Can you work these out from the model? Positions are in its coordinate system, mm. A direction names the side the tool comes from. Give positions to 0.01 mm unless a question says otherwise; leave off trailing zeros. Write each loop counter-clockwise with the first axis right and the second up, starting at its lowest first coordinate (ties: lowest second). Pieces come first, ordered by that corner, then holes.
```python
from build123d import *

# Parameters (mm, degrees)
F0_R     = 3.875
F1_DEPTH = 3
F0_R_2   = 7
F2_DEPTH = 0.6
F0_R_3   = 11.5
F3_DEPTH = 2
F4_DEPTH = 2
F6_T     = 1


# Not quite as in the source:
# - a shell that OpenCascade refuses in one call is made with other operations: the cavity is built on its own and cut out
# - the program builds the solid bodies; features that only make, move or delete a surface that nothing else refers to are left out


with BuildPart() as f1:
    # F0 (on Top) → F1 (new body)
    with BuildSketch(Plane.XY):
        Circle(F0_R)
    extrude(amount=F1_DEPTH)

    # F0 (on Top) → F2 (join)
    with BuildSketch(Plane.XY):
        Circle(F0_R_2)
        Circle(F0_R, mode=Mode.SUBTRACT)
    extrude(amount=F2_DEPTH)

    # F0 (on Top) → F3 (join)
    with BuildSketch(Plane.XY):
        Circle(F0_R_3)
        Circle(F0_R_2, mode=Mode.SUBTRACT)
        Circle(F0_R_2)
        Circle(F0_R, mode=Mode.SUBTRACT)
    extrude(amount=-F3_DEPTH)

    # F0 (on Top) → F4 (join)
    with BuildSketch(Plane.XY):
        Circle(F0_R)
    extrude(amount=-F4_DEPTH)

    # F6: shell of thickness 1, made by hand


with BuildPart() as f6_core1:
    # F6_t2: copy of F1
    add(f1.part)

    # the walls: a layer under each face that stays
    f6_faces = [f6_core1.faces().sort_by_distance(p)[0] for p in [
        (-3.875, 0, 1.8),
        (-4.6666666667, -4.6666666667, 0.6),
        (-7, 0, 0.3),
        (-7.6666666667, -7.6666666667, 0),
        (-11.5, 0, -1),
        (0, 0, -2),
    ]]
    thicken(f6_faces, amount=-F6_T, mode=Mode.SUBTRACT)

    # F6_s3 → F6_t4 (revolve, cut)
    with BuildSketch(Plane.XZ):
        Polygon((3.885, 0.61), (2.875, 0.6), (2.875, -0.4), (3.875, -0.4), align=None)
    revolve(axis=Axis((0, 0, 0.6), (0, 0, 1)), mode=Mode.SUBTRACT)

    # F6_s5 → F6_t6 (revolve, cut)
    with BuildSketch(Plane.XZ):
        Polygon((7.01, 0.01), (6, 0), (6, -1), (7, -1), align=None)
    revolve(axis=Axis((0, 0, 0), (0, 0, 1)), mode=Mode.SUBTRACT)


with BuildPart() as f1_1:
    add(f1.part)

    # what is left inside the walls is the cavity
    f6_cavity = [f6_core1.part.solids().sort_by_distance(p)[0] for p in [
        (0, -2, -0.99),
    ]]
    add(f6_cavity, mode=Mode.SUBTRACT)


solid = f1_1.part
```
1) Suppose I cut it at A-A on x = 0. Write out the boundary of the cut face in (y, z) (3 decimals), plus the area to 4 significant figures.
Values follow:
outline: (-11.5, -2) - (11.5, -2) - (11.5, 0) - (7, 0) - (7, 0.6) - (3.875, 0.6) - (3.875, 3) - (2.875, 3) - (2.875, -0.4) - (6, -0.4) - (6, -1) - (-6, -1) - (-6, -0.4) - (-2.875, -0.4) - (-2.875, 3) - (-3.875, 3) - (-3.875, 0.6) - (-7, 0.6) - (-7, 0) - (-11.5, 0) - close
area: 46.25 mm2
2) Suppose I cut it at C-C on z = 1.7. Write out the boundary of the cut face in (x, y) (3 decimals), plus the area to 3 significant figures.
Values follow:
outline: circle Ø7.75 at (0, 0); hole circle Ø5.75 at (0, 0)
area: 21.2 mm2
3) For faces 1 (the face through (-1, 3, 3)), 2 (the face through (6.466, -2.681, 0.296)), 3 (the face through (0, 0, -1)), which set-ups out of +Z, -Z, +X, -X, +Y, -Y let a thin tool reach every point of the face, with its end or its side?
Values follow:
face 1: +Z, +X, -X, +Y, -Y
face 2: +Z
face 3: none
4) Suppose I cut it at B-B on y = 5. Write out the boundary of the cut face in (x, z), plus the area to 3 significant figures.
Values follow:
outline: (-10.36, -2) - (10.36, -2) - (10.36, 0) - (4.9, 0) - (4.9, 0.6) - (-4.9, 0.6) - (-4.9, 0) - (-10.36, 0) - close; hole (-3.32, -1) - (3.32, -1) - (3.32, -0.4) - (-3.32, -0.4) - close
area: 43.3 mm2
5) For pin 1 Ø1.5 at (x, z) = (2.5, -0.5) entering from +Y; pin 2 Ø2 at (x, y) = (2, -7.5) entering from +Z; pin 3 Ø5 at (x, y) = (0, 0) entering from +Z, each with a flat end and sliding along its axis, tell me the tip position at first contact or that it passes through.
Values follow:
pin 1: stops at y = 11.37
pin 2: stops at z = 0.6
pin 3: stops at z = -1
6) If we mould it in two halves opening along Z, with no side actions, what happens to faces 4 (the face through (-1.5, 11.4, -1)), 5 (the face through (3, 1, -0.4)), 6 (the face through (-5.994, 0.264, -0.704)), 7 (the face through (0, 0, -2))? For each: +Z half, -Z half, draft (parallel to the pull), parting line (faces both ways), or undercut.
Values follow:
face 4: draft
face 5: undercut
face 6: undercut
face 7: -Z half
7) Please list where these lines run through material, in increasing order: L1, parallel to Y at x = 0, z = -0.75; L2, parallel to Z at x = -2.5, y = 2.5; L3, parallel to Z at x = -1.5, y = -4.
Values follow:
L1: y = -11.5 to -6, 6 to 11.5
L2: z = -2 to -1, -0.4 to 3
L3: z = -2 to -1, -0.4 to 0.6
8) Suppose I cut it at D-D on x = 5.25. Write out the boundary of the cut face in (y, z), plus the area to 3 significant figures.
Values follow:
outline: (-10.23, -2) - (10.23, -2) - (10.23, 0) - (4.63, 0) - (4.63, 0.6) - (-4.63, 0.6) - (-4.63, 0) - (-10.23, 0) - close; hole (-2.9, -1) - (2.9, -1) - (2.9, -0.4) - (-2.9, -0.4) - close
area: 43.0 mm2
